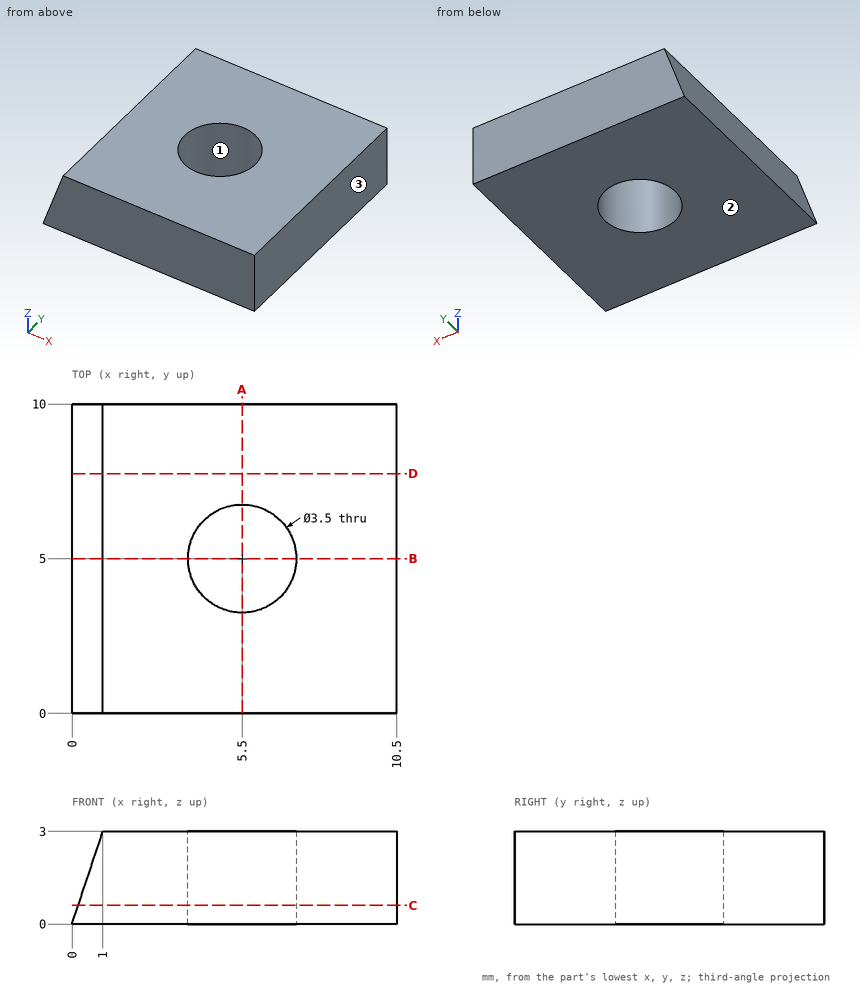
Geometry: see drawing. Coordinates: mm, zero at the bounding-box minimum. Give positions to 0.01 mm unless a question says otherwise; leave off trailing zeros. Loops run counter-clockwise (first coordinate to the right, second up) from the corner with the lowest first, then second, coordinate; pieces in that order, holes last. Notation, with made-up numbers: (-19, -17.75) -> (8, -17.75) arc R20 cw to (8, 2.25) -> close; hole circle Ø10 at (63, 18). An arc over 180 degrees is marked (long way). Answer as a JSON object with one key per item and string values. Group by question number.
Item 1: Line query: probe 1 along Y at (x, z) = (5.5, 1.5); probe 2 along X at (y, z) = (3.75, 1.95); probe 3 along X at (y, z) = (7.5, 2). Output: solid intervals per line, ascending.
Item 2: Cut plane B-B, the plane y = 5. Return the cut outline in (x, z), and give its area (3 significant figures).
Item 3: Cut plane D-D, the plane y = 7.75. Return the cut outline in (x, z).
Item 4: Cut plane A-A, the plane x = 5.5. Return the cut outline in (y, z), and give its area (3 significant figures).
Item 5: Cut plane C-C, the plane z = 0.6. Return the cut outline in (x, y), and give its area (3 significant figures).
Item 6: Pin query (flat end, axial travel): P1, Ø4.5, axis at x = 5.5, y = 5, coming from the +Z side. Return the tip coordinate at first contact, or that it passes through.
Item 7: Pull-direction query (X, two-part tool) for the marked faces 1, 2 and 3; classes: released by +X, released by -X, zero draft, split by the parting line, or undercut.
Checks:
{
 "1": {"probe 1": "y = 0 to 3.25, 6.75 to 10", "probe 2": "x = 0.65 to 4.28, 6.72 to 10.5", "probe 3": "x = 0.67 to 10.5"},
 "2": {"outline": "(0, 0) -> (3.75, 0) -> (3.75, 3) -> (1, 3) -> close; (7.25, 0) -> (10.5, 0) -> (10.5, 3) -> (7.25, 3) -> close", "area": "19.5 mm²"},
 "3": {"outline": "(0, 0) -> (10.5, 0) -> (10.5, 3) -> (1, 3) -> close"},
 "4": {"outline": "(0, 0) -> (3.25, 0) -> (3.25, 3) -> (0, 3) -> close; (6.75, 0) -> (10, 0) -> (10, 3) -> (6.75, 3) -> close", "area": "19.5 mm²"},
 "5": {"outline": "(0.2, 0) -> (10.5, 0) -> (10.5, 10) -> (0.2, 10) -> close; hole circle Ø3.5 at (5.5, 5)", "area": "93.4 mm²"},
 "6": {"P1": "stops at z = 3"},
 "7": {"face 1": "undercut", "face 2": "zero draft", "face 3": "released by +X"}
}
